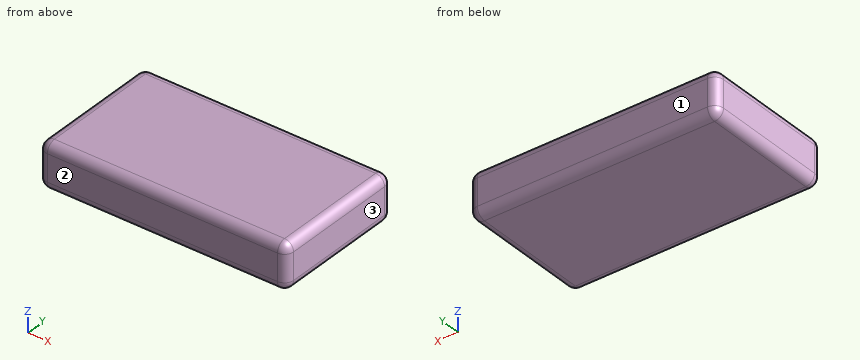
```python
from build123d import *

# Parameters (mm, degrees)
F0_W     = 55
F0_H     = 30
F1_DEPTH = 10
F2_R     = 2
F3_R     = 2


with BuildPart() as f1:
    # F0 (on Top) → F1 (new body)
    with BuildSketch(Plane.XY):
        Rectangle(F0_W, F0_H)
    extrude(amount=F1_DEPTH)

    # F2
    f2_edges = [f1.edges().sort_by_distance(p)[0] for p in [
        (27.5, 0, 0),
        (27.5, 0, 10),
    ]]
    fillet(f2_edges, radius=F2_R)

    # F3
    f3_edges = [f1.edges().sort_by_distance(p)[0] for p in [
        (-27.5, 0, 10),
        (-27.5, 0, 0),
        (-27.5, -15, 5),
        (27.5, -15, 5),
        (27.5, 15, 5),
        (26.914214, 15, 0.585786),
        (26.914214, 15, 9.414214),
        (-1, 15, 0),
        (-1, 15, 10),
        (-27.5, 15, 5),
    ]]
    fillet(f3_edges, radius=F3_R)


solid = f1.part
```
Geometry check sheet. Reference: the model listing, model coordinates, mm. Face numbers are marked on the shaded views. Give positions to 0.01 mm unless a question says otherwise; leave off trailing zeros. Order: outer loops, then holes, each group sorted by start corner. A loop starts at its lowest first (then second) coordinate and runs counter-clockwise, first axis right, second up. Notation, with made-up numbers: (78, -4.5) - (102, -4.5) arc R23 cw to (102, 22.5) - close; hole circle Ø11 at (30.5, -39). An arc over 180 degrees is marked (long way). Write item = value, one per line. Start each with the question number.
1) Scan lines: L1, parallel to Z at x = 6, y = 13.25; L2, parallel to Y at x = 13.5, z = 9; L3, parallel to Y at x = 21.5, z = 8.25. Record each from-to range of solid material in increasing order.
2) Draft check along Y on the marked faces 1, 2 and 3. Enter one of: released by +Y, released by -Y, zero draft, split by the parting line, or undercut.
3) Section check A-A (z = 1). Enter the section's corners in (x, y), then the cut area to 3 significant figures.
Geometry check:
q1.L1 = 0.02 to 9.98
q1.L2 = -14.73 to 14.73
q1.L3 = -14.98 to 14.98
q2.face_1 = released by +Y
q2.face_2 = released by -Y
q2.face_3 = zero draft
q3.outline = (-27.23, -13) arc R1.73 ccw to (-25.5, -14.73) - (25.5, -14.73) arc R1.73 ccw to (27.23, -13) - (27.23, 13) arc R1.73 ccw to (25.5, 14.73) - (-25.5, 14.73) arc R1.73 ccw to (-27.23, 13) - close
q3.area = 1,600 mm2
